```python
from build123d import *

# Parameters (mm, degrees)
SKETCH1_R                = 15
BOSS_EXTRUDE1_DEPTH      = 40
SKETCH2_R                = 30
BOSS_EXTRUDE2_DEPTH      = 5
CHAMFER1_SIZE            = 2
FILLET1_R                = 3
SKETCH3_R                = 2.5
CUT_EXTRUDE1_DEPTH       = 96
CIRPATTERN2_COUNT        = 6
MIRROR1_COPY_1_SKETCH_R  = 2.5
MIRROR1_COPY_1_DEPTH     = 96
MIRROR1_COPY_2_SKETCH_R  = 2.5
MIRROR1_COPY_2_DEPTH     = 96
MIRROR1_COPY_3_SKETCH_R  = 2.5
MIRROR1_COPY_3_DEPTH     = 96
MIRROR1_COPY_4_SKETCH_R  = 2.5
MIRROR1_COPY_4_DEPTH     = 96
MIRROR1_COPY_5_SKETCH_R  = 2.5
MIRROR1_COPY_5_DEPTH     = 96
CHAMFER1_OF_MIRROR1_SIZE = 2
FILLET1_OF_MIRROR1_R     = 3


with BuildPart() as part:
    # Sketch1 → Boss-Extrude1 (new, symmetric)
    with BuildSketch(Plane(origin=(0, 0, 0), x_dir=(1, 0, 0), z_dir=(0, 1, 0))):
        with Locations(Location((-0.757761668, 0, 0), (0, 0, 270))):
            Circle(SKETCH1_R)
    extrude(amount=BOSS_EXTRUDE1_DEPTH, both=True)

    # Sketch2 → Boss-Extrude2 (add)
    with BuildSketch(Plane(origin=(0, 40, 0), x_dir=(1, 0, 0), z_dir=(0, 1, 0))):
        with Locations(Location((0, 0, 0), (0, 0, 270))):
            Circle(SKETCH2_R)
    boss_extrude2 = extrude(amount=BOSS_EXTRUDE2_DEPTH)

    # Chamfer1
    chamfer1_edges = [part.edges().sort_by_distance(p)[0] for p in [
        (0, 40, -30),
        (0, 45, -30),
    ]]
    chamfer(chamfer1_edges, length=CHAMFER1_SIZE)

    # Fillet1
    fillet1_edges = [part.edges().sort_by_distance(p)[0] for p in [
        (0, 40, -28),
    ]]
    fillet(fillet1_edges, radius=FILLET1_R)

    # Sketch3 → Cut-Extrude1 (cut, through all)
    with BuildSketch(Plane(origin=(0, 45, 0), x_dir=(1, 0, 0), z_dir=(0, 1, 0))):
        with Locations(Location((-0.378880834, 21.5, 0), (0, 0, 270))):
            Circle(SKETCH3_R)
    cut_extrude1 = extrude(amount=-CUT_EXTRUDE1_DEPTH, mode=Mode.SUBTRACT)

    # CirPattern2: Cut-Extrude1 ×6 about axis
    cirpattern2_axis = Axis((0, 0, 0), (0, 1, 0))
    for i in range(1, CIRPATTERN2_COUNT):
        add(cut_extrude1.rotate(cirpattern2_axis, i * 360 / CIRPATTERN2_COUNT), mode=Mode.SUBTRACT)

    # Sketch5 → CBORE for M12 Hex Head Bolt1 (revolve, cut)
    with BuildSketch(Plane(origin=(0, 45, 0), x_dir=(0, 0, 1), z_dir=(1, 0, 0))):
        Polygon((0, 0), (0, 90), (6.75, 90), (6.75, 7.95), (11.89, 7.95), (11.89, 0.025), (11.915, 0), align=None)
    cbore_for_m12_hex_head_bolt1 = revolve(axis=Axis((0, 51.35, 0), (0, -1, 0)), mode=Mode.SUBTRACT)

    # Mirror1: Boss-Extrude2, Cut-Extrude1, CBORE for M12 Hex Head Bolt1 across plane
    add(boss_extrude2.mirror(Plane.ZX))
    add(cut_extrude1.mirror(Plane.ZX), mode=Mode.SUBTRACT)
    add(cbore_for_m12_hex_head_bolt1.mirror(Plane.ZX), mode=Mode.SUBTRACT)

    # Mirror1 copy 1 sketch → Mirror1 copy 1 (cut, through all)
    with BuildSketch(Plane(origin=(0, -45, 0), x_dir=(0.5000000000000001, 0, -0.8660254037844386), z_dir=(0, -1, 0))):
        with Locations((-0.378880834, -21.5)):
            Circle(MIRROR1_COPY_1_SKETCH_R)
    extrude(amount=-MIRROR1_COPY_1_DEPTH, mode=Mode.SUBTRACT)

    # Mirror1 copy 2 sketch → Mirror1 copy 2 (cut, through all)
    with BuildSketch(Plane(origin=(0, -45, 0), x_dir=(-0.4999999999999998, 0, -0.8660254037844387), z_dir=(0, -1, 0))):
        with Locations((-0.378880834, -21.5)):
            Circle(MIRROR1_COPY_2_SKETCH_R)
    extrude(amount=-MIRROR1_COPY_2_DEPTH, mode=Mode.SUBTRACT)

    # Mirror1 copy 3 sketch → Mirror1 copy 3 (cut, through all)
    with BuildSketch(Plane(origin=(0, -45, 0), x_dir=(-1, 0, 0), z_dir=(0, -1, 0))):
        with Locations((-0.378880834, -21.5)):
            Circle(MIRROR1_COPY_3_SKETCH_R)
    extrude(amount=-MIRROR1_COPY_3_DEPTH, mode=Mode.SUBTRACT)

    # Mirror1 copy 4 sketch → Mirror1 copy 4 (cut, through all)
    with BuildSketch(Plane(origin=(0, -45, 0), x_dir=(-0.5000000000000004, 0, 0.8660254037844384), z_dir=(0, -1, 0))):
        with Locations((-0.378880834, -21.5)):
            Circle(MIRROR1_COPY_4_SKETCH_R)
    extrude(amount=-MIRROR1_COPY_4_DEPTH, mode=Mode.SUBTRACT)

    # Mirror1 copy 5 sketch → Mirror1 copy 5 (cut, through all)
    with BuildSketch(Plane(origin=(0, -45, 0), x_dir=(0.5000000000000001, 0, 0.8660254037844386), z_dir=(0, -1, 0))):
        with Locations((-0.378880834, -21.5)):
            Circle(MIRROR1_COPY_5_SKETCH_R)
    extrude(amount=-MIRROR1_COPY_5_DEPTH, mode=Mode.SUBTRACT)

    # Chamfer1 of Mirror1
    chamfer1_of_mirror1_edges = [part.edges().sort_by_distance(p)[0] for p in [
        (0, -40, -30),
        (0, -45, -30),
    ]]
    chamfer(chamfer1_of_mirror1_edges, length=CHAMFER1_OF_MIRROR1_SIZE)

    # Fillet1 of Mirror1
    fillet1_of_mirror1_edges = [part.edges().sort_by_distance(p)[0] for p in [
        (0, -40, -28),
    ]]
    fillet(fillet1_of_mirror1_edges, radius=FILLET1_OF_MIRROR1_R)


solid = part.part
```
CAD build for the part. Positions are in the model's coordinates, mm. A direction names the side the tool comes from. Round coordinates to 2 decimals unless told otherwise and drop trailing zeros. Write each loop counter-clockwise with the first axis right and the second up, starting at its lowest first coordinate (ties: lowest second). Pieces come first, ordered by that corner, then holes.
Item 1: Drop flat-ended pins along their axis: pin 1 Ø1 at (y, z) = (-30, 6) entering from +X; pin 2 Ø3 at (x, z) = (-18.81, -10.42) entering from -Y; pin 3 Ø8 at (x, z) = (0.38, 21.5) entering from +Y; pin 4 Ø12 at (y, z) = (-5, -13.5) entering from +X. Give the stop position or say it passes through.
Filled in:
pin 1: stops at x = 13.2
pin 2: passes through
pin 3: stops at y = 45
pin 4: stops at x = 12.23
Item 2: Drill centre lines: L1, parallel to Y at x = -20, z = -15; L2, parallel to X at y = 43, z = 0; L3, parallel to X at y = -26, z = 6. Where is each one in solid material? Low to high.
Filled in:
L1: y = -45 to -40, 40 to 45
L2: x = -30 to -11.89, 11.89 to 30
L3: x = -14.51 to -3.09, 3.09 to 12.99
Item 3: Tool access for faces 1 (the cylindrical face through (-19.56, 42.535, -12.806)), 2 (the cylindrical face through (11.607, 41.068, -2.578)), 3 (the flat face through (5, -37.05, -5)): list every direction of +Z, -Z, +X, -X, +Y, -Y with a clear straight run to the whole face (end or side of a thin tool).
Filled in:
face 1: +Y, -Y
face 2: +Y
face 3: -Y
Item 4: Band-saw the part on B-B on y = 14. Write the cut outline in (x, z).
Filled in:
outline: circle Ø30 at (-0.76, 0); hole circle Ø13.5 at (0, 0)
Item 5: Band-saw the part on A-A on z = 21.5. Give the number of separate pieces and of enclosed holes in the cut face, then the cut area to 3 significant figures.
Filled in:
separate pieces: 4
enclosed holes: 0
area: 344 mm2
Item 6: Mould opens along X. For faces 4 (the cylindrical face through (0.7, -42.54, 19.02)), 5 (the flat face through (-12, -40, 12)), 6 (the cylindrical face through (-0.098, 0.56, -14.985)) say: released by +X, released by -X, zero draft, split by the parting line, or undercut.
Filled in:
face 4: undercut
face 5: zero draft
face 6: split by the parting line
